Geometry: final body of the model. Coordinates: model frame, mm. A direction names the side the tool comes from. Round coordinates to 2 decimals unless told otherwise and drop trailing zeros. Loops run counter-clockwise (first coordinate to the right, second up) from the corner with the lowest first, then second, coordinate; pieces in that order, holes last. Notation, with made-up numbers: (33, 35) - (53, 35) arc R22 ccw to (53, 41) - close; hole circle Ø1 at (66, -24.5). An arc over 180 degrees is marked (long way). Write item = value, one per line. Start each with the question number.
Item 1: First-contact query: pin 1 (2 mm diameter, centred on x = 18, y = 7.5, fed in from +Z); pin 2 (3 mm diameter, centred on x = 12.5, y = 4, fed in from -Z); pin 3 (3.5 mm diameter, centred on x = 6.5, y = 5.5, fed in from -Z). Flat tips, straight axial feed; report the tip coordinate or a pass-through.
Item 2: Section A-A (x = 13.5). Return loops of the section in (y, z), plus the area to 3 significant figures.
Item 3: Access query for faces 3 (the flat face through (12, 6, 0.25)), 4 (the flat face through (24, -2, -2)). Directions: +Z, -Z, +X, -X, +Y, -Y. A direction counts if a zero-diameter tool reaches every point of the face in a straight line with its end or side. Return the directions, or none.
Item 4: Draft query along Z for faces 1 (the cylindrical face through (12.2, -2.5, 0.1)), 2 (the flat face through (0, -2, -2)). Return one class per face: pulls with the +Z half, pulls with the -Z half, needs draft (parallel to the pull), parting line crosses it, or undercut.
Item 5: Line query: line 1 (Z direction, x = 6, y = 0); line 2 (Y direction, x = 14.5, z = 0); line 3 (Z direction, x = 6.25, y = 5.5). Output: solid intervals per line, ascending. Write a range as from..to.
from build123d import *

# Parameters (mm, degrees)
SKETCH1_R           = 9.7
BOSS_EXTRUDE1_DEPTH = 24
SKETCH2_R           = 2.5
CUT_EXTRUDE1_DEPTH  = 28.643805816
SKETCH3_W           = 0.5
SKETCH3_H           = 19.4
CUT_EXTRUDE2_DEPTH  = 28.643805816
CHAMFER1_SIZE       = 0.8


with BuildPart() as part:
    # Sketch1 → Boss-Extrude1 (new body)
    with BuildSketch(Plane(origin=(0, 0, 0), x_dir=(0, 0, -1), z_dir=(1, 0, 0))):
        Circle(SKETCH1_R)
    extrude(amount=BOSS_EXTRUDE1_DEPTH)

    # Sketch2 → Cut-Extrude1 (cut, through all)
    with BuildSketch(Plane(origin=(24, 0, 0), x_dir=(0, 0, -1), z_dir=(1, 0, 0))):
        Circle(SKETCH2_R)
    extrude(amount=-CUT_EXTRUDE1_DEPTH, mode=Mode.SUBTRACT)

    # Sketch3 → Cut-Extrude2 (cut, through all)
    with BuildSketch(Plane.ZY):
        with Locations((0, 9.7)):
            Rectangle(SKETCH3_W, SKETCH3_H)
    extrude(amount=-CUT_EXTRUDE2_DEPTH, mode=Mode.SUBTRACT)

    # Chamfer1
    chamfer1_edges = [part.edges().sort_by_distance(p)[0] for p in [
        (0, -6.946761836, 6.769970458),
        (24, -6.946761836, 6.769970458),
    ]]
    chamfer(chamfer1_edges, length=CHAMFER1_SIZE)


solid = part.part
Taken from the geometry:
q1.pin_1 = 7.2
q1.pin_2 = -9.37
q1.pin_3 = -8.95
q2.outline = (2.49, -0.25) arc R2.5 cw (long way) to (2.49, 0.25) - (9.7, 0.25) arc R9.7 ccw (long way) to (9.7, -0.25) - close
q2.area = 272 mm^2
q3.face_3 = +X, -X, +Y
q3.face_4 = +Z, -Z, +X, +Y, -Y
q4.face_1 = undercut
q4.face_2 = needs draft
q5.line_1 = -9.7..-2.5, 2.5..9.7
q5.line_2 = -9.7..-2.5
q5.line_3 = -7.99..-0.25, 0.25..7.99
